Verification items for the finished model (mm, model axes). A direction names the side the tool comes from. Give positions to 0.01 mm unless a question says otherwise; leave off trailing zeros. Write each loop counter-clockwise with the first axis right and the second up, starting at its lowest first coordinate (ties: lowest second). Pieces come first, ordered by that corner, then holes. Notation, with made-up numbers: (29.25, 53) -> (37.25, 53) arc R20 ccw to (37.25, 84) -> close; hole circle Ø5 at (-32, 4). An arc over 180 degrees is marked (long way). Write item = value, one per line.
from build123d import *

# Parameters (mm, degrees)
SKETCH1_W           = 15.8
SKETCH1_H           = 3.2
BOSS_EXTRUDE1_DEPTH = 7.8
SHELL1_T            = -1.2
SKETCH3_W           = 15.8
SKETCH3_H           = 1.65
CUT_EXTRUDE1_DEPTH  = 1.1
LPATTERN1_COUNT     = 2
LPATTERN1_PITCH     = 3.15
SKETCH5_W           = 13.4
SKETCH5_H           = 1.65
CUT_EXTRUDE2_DEPTH  = 18.74514018
LPATTERN2_COUNT     = 2
LPATTERN2_PITCH     = 3.15
SKETCH7_W           = 3
SKETCH7_H           = 1.5
BOSS_EXTRUDE2_DEPTH = 1.8


with BuildPart() as part:
    # Sketch1 → Boss-Extrude1 (new body)
    with BuildSketch(Plane.XY):
        with Locations((7.9, 1.6)):
            Rectangle(SKETCH1_W, SKETCH1_H)
    extrude(amount=-BOSS_EXTRUDE1_DEPTH)

    # Shell1
    shell1_openings = [part.faces().sort_by_distance(p)[0] for p in [
        (7.9, 0, -3.9),
    ]]
    offset(amount=SHELL1_T, openings=shell1_openings, kind=Kind.INTERSECTION)

    # Sketch3 → Cut-Extrude1 (cut)
    with BuildSketch(Plane(origin=(0, 3.2, 0), x_dir=(1, 0, 0), z_dir=(0, 1, 0))):
        with Locations((7.9, 5.475)):
            Rectangle(SKETCH3_W, SKETCH3_H)
    cut_extrude1 = extrude(amount=-CUT_EXTRUDE1_DEPTH, mode=Mode.SUBTRACT)

    # LPattern1: Cut-Extrude1 ×2
    with Locations(*[(0, 0, i * LPATTERN1_PITCH) for i in range(1, LPATTERN1_COUNT)]):
        add(cut_extrude1, mode=Mode.SUBTRACT)

    # Sketch5 → Cut-Extrude2 (cut, through all)
    with BuildSketch(Plane(origin=(0, 2.1, 0), x_dir=(1, 0, 0), z_dir=(0, 1, 0))):
        with Locations((7.9, 5.475)):
            Rectangle(SKETCH5_W, SKETCH5_H)
    cut_extrude2 = extrude(amount=-CUT_EXTRUDE2_DEPTH, mode=Mode.SUBTRACT)

    # LPattern2: Cut-Extrude2 ×2
    with Locations(*[(0, 0, i * LPATTERN2_PITCH) for i in range(1, LPATTERN2_COUNT)]):
        add(cut_extrude2, mode=Mode.SUBTRACT)

    # Sketch7 → Boss-Extrude2 (add)
    with BuildSketch(Plane.XZ.offset(-2)):
        with Locations((7.9, -3.9)):
            Rectangle(SKETCH7_W, SKETCH7_H)
    extrude(amount=BOSS_EXTRUDE2_DEPTH)


solid = part.part
Item 1: Sectioned sample at B-B on z = -5.25. Record the cut outline in (x, y).
Response values:
outline = (0, 0) -> (1.2, 0) -> (1.2, 2.1) -> (0, 2.1) -> close; (14.6, 0) -> (15.8, 0) -> (15.8, 2.1) -> (14.6, 2.1) -> close
Item 2: Sectioned sample at D-D on z = -4. Record the cut outline in (x, y).
Response values:
outline = (0, 0) -> (1.2, 0) -> (1.2, 2) -> (6.4, 2) -> (6.4, 0.2) -> (9.4, 0.2) -> (9.4, 2) -> (14.6, 2) -> (14.6, 0) -> (15.8, 0) -> (15.8, 3.2) -> (0, 3.2) -> close
Item 3: Go/stop test with flat-tipped pins: P1, Ø4, axis at x = 11, z = -3.5, coming from the -Y side; P2, Ø1, axis at x = 1, z = -5.5, coming from the +Y side. Record where each tip stops, or that it passes through.
Response values:
P1 = 0.2
P2 = 2.1
Item 4: Sectioned sample at A-A on x = 11.5. Record the cut outline in (y, z).
Response values:
outline = (0, -7.8) -> (3.2, -7.8) -> (3.2, -6.3) -> (2, -6.3) -> (2, -6.6) -> (0, -6.6) -> close; (0, -1.2) -> (2, -1.2) -> (2, -1.5) -> (3.2, -1.5) -> (3.2, 0) -> (0, 0) -> close; (2, -4.65) -> (3.2, -4.65) -> (3.2, -3.15) -> (2, -3.15) -> close
Item 5: Set-up check for faces 1 (the flat face through (8, 3.2, -4)), 2 (the flat face through (15, 2.1, -5)), 3 (the flat face through (9.4, 1, -4)), 4 (the flat face through (8, 2, -3.15)): record each of +Z, -Z, +X, -X, +Y, -Y from which the full face is reachable in a straight line by a thin tool's end or side.
Response values:
face_1 = +Z, -Z, +X, -X, +Y
face_2 = +X, -X, +Y
face_3 = -Y
face_4 = +Y
Item 6: Material ranges on line 1 (Z direction, x = 8.5, y = 0.95); line 2 (Z direction, x = 5.5, y = 2.05); line 3 (Z direction, x = 12, y = 0.2), recorded low to high.
Response values:
line_1 = -7.8 to -6.6, -4.65 to -3.15, -1.2 to 0
line_2 = -7.8 to -6.3, -4.65 to -3.15, -1.5 to 0
line_3 = -7.8 to -6.6, -1.2 to 0
Item 7: Sectioned sample at C-C on y = 0.65. Record the cut outline in (x, z), then the cut area to 3 significant figures.
Response values:
outline = (0, -7.8) -> (15.8, -7.8) -> (15.8, 0) -> (0, 0) -> close; (6.4, -4.65) -> (9.4, -4.65) -> (9.4, -3.15) -> (6.4, -3.15) -> close; hole (1.2, -6.6) -> (14.6, -6.6) -> (14.6, -1.2) -> (1.2, -1.2) -> close
area = 55.4 mm^2
